from build123d import *

# Parameters (mm, degrees)
SKETCH1_W           = 480
SKETCH1_H           = 480
BOSS_EXTRUDE1_DEPTH = 190
BOSS_EXTRUDE1_DRAFT = 20
FILLET1_R           = 20
SKETCH2_R           = 120
BOSS_EXTRUDE2_DEPTH = 30
BOSS_EXTRUDE2_TAPER = 20
SHELL1_T            = -10
SCALE1_SCALE        = 0.5


with BuildPart() as part:
    # Sketch1 → Boss-Extrude1 (with draft: the straight prism first)
    with BuildSketch(Plane(origin=(0, 0, 0), x_dir=(1, 0, 0), z_dir=(0, 1, 0))):
        with Locations((240, -240)):
            Rectangle(SKETCH1_W, SKETCH1_H)
    extrude(amount=-BOSS_EXTRUDE1_DEPTH)
    # Boss-Extrude1: the draft: its side faces are tilted about the plane it starts from
    boss_extrude1_sides = [part.faces().sort_by_distance(p)[0] for p in [
        (0, -95, 240),
        (240, -95, 480),
        (480, -95, 240),
        (240, -95, 0),
    ]]
    draft(boss_extrude1_sides, Plane(origin=(0, 0, 0), x_dir=(1, 0, 0), z_dir=(0, 1, 0)), BOSS_EXTRUDE1_DRAFT)

    # Fillet1
    fillet1_edges = [part.edges().sort_by_distance(p)[0] for p in [
        (549.154344511, -190, 240),
        (240, -190, -69.154344511),
        (-69.154344511, -190, 240),
        (240, 0, 0),
        (480, 0, 240),
        (240, 0, 480),
        (0, 0, 240),
        (-34.577172255, -95, -34.577172255),
        (514.577172255, -95, -34.577172255),
        (514.577172255, -95, 514.577172255),
        (-34.577172255, -95, 514.577172255),
        (240, -190, 549.154344511),
    ]]
    fillet(fillet1_edges, radius=FILLET1_R)

    # Sketch2 → Boss-Extrude2 (add)
    with BuildSketch(Plane(origin=(0, 0, 0), x_dir=(1, 0, 0), z_dir=(0, 1, 0))):
        with Locations((240, -240)):
            Circle(SKETCH2_R)
    extrude(amount=BOSS_EXTRUDE2_DEPTH, taper=BOSS_EXTRUDE2_TAPER)

    # Shell1
    shell1_openings = [part.faces().sort_by_distance(p)[0] for p in [
        (240, 30, 240),
    ]]
    offset(amount=SHELL1_T, openings=shell1_openings, kind=Kind.INTERSECTION)


with BuildPart() as part_1:
    # Scale1: scaled about (0, 0, 0)
    add(part.part.scale(SCALE1_SCALE))


solid = part_1.part
Verification items for the finished model (mm, model axes). A direction names the side the tool comes from. Coordinates: 2 decimals unless noted, no trailing zeros. Write each loop counter-clockwise with the first axis right and the second up, starting at its lowest first coordinate (ties: lowest second). Pieces come first, ordered by that corner, then holes. Notation, with made-up numbers: M 45.5,19 L 103.5,19 A33 ccw 103.5,58 Z; hole C -29,6.25 d9. An arc over 180 degrees is marked long. Use a Markdown table: item, result.
Q1. Sectioned sample at C-C, the plane y = 6.5. Record the boundary of the cut face in (x, z).
Reply:
| item | result |
|---|---|
| outline | C 120,120 d115.27; hole C 120,120 d104.63 |
Q2. Sectioned sample at D-D, the plane x = 120. Record the boundary of the cut face in (y, z), plus the area to 3 significant figures.
Reply:
| item | result |
|---|---|
| outline | M -95,-20.3 A10 ccw -81.58,-29.69 L -6.58,-2.39 A10 ccw 0,7 L 0,60 L 15,65.46 L 15,70.78 L -5,63.5 L -5,7 A5 cw -8.29,2.3 L -83.29,-24.99 A5 cw -90,-20.3 L -90,260.3 A5 cw -83.29,264.99 L -8.29,237.7 A5 cw -5,233 L -5,176.5 L 15,169.22 L 15,174.54 L 0,180 L 0,233 A10 ccw -6.58,242.39 L -81.58,269.69 A10 ccw -95,260.3 Z |
| area | 3,170 mm² |
Q3. Go/stop test with flat-tipped pins: P1, Ø12, axis at x = 179, z = 85, coming from the +Y side; P2, Ø8, axis at y = -63.5, z = 14.5, coming from the -X side; P3, Ø5, axis at x = 82, y = -2.5, coming from the +Z side. Record where each tip stops, or that it passes through.
Reply:
| item | result |
|---|---|
| P1 | stops at y = 0 |
| P2 | stops at x = -24.57 |
| P3 | stops at z = 241.66 |
Q4. Sectioned sample at A-A, the plane z = 45. Record the boundary of the cut face in (x, y), plus the area to 3 significant figures.
Reply:
| item | result |
|---|---|
| outline | M -29.69,-81.58 A10 ccw -20.3,-95 L 260.3,-95 A10 ccw 269.69,-81.58 L 242.39,-6.58 A10 ccw 233,0 L 7,0 A10 ccw -2.39,-6.58 Z; hole M -24.99,-83.29 A5 ccw -20.3,-90 L 260.3,-90 A5 ccw 264.99,-83.29 L 237.7,-8.29 A5 ccw 233,-5 L 7,-5 A5 ccw 2.3,-8.29 Z |
| area | 3,570 mm² |
Q5. Thickness scan on line 1 (Y direction, x = 179.5, z = 178.5); line 2 (Z direction, x = 203, y = -36.5); line 3 (Z direction, x = 140.5, y = -89). Record the ranges inside material, lowest first.
Reply:
| item | result |
|---|---|
| line 1 | y = -95 to -90, -5 to 0 |
| line 2 | z = -13.28 to -7.96, 247.96 to 253.28 |
| line 3 | z = -29.46 to -23.3, 263.3 to 269.46 |
Q6. Draft check along Z on faces 1 (the face through (-15.85, -43.55, 121.96)), 2 (the face through (-13.2, -43.45, 253.05)), 3 (the face through (-24.43, -87.81, 118.04)). Enter one of: +Z half, -Z half, draft (parallel to the pull), parting line (faces both ways), or undercut.
Reply:
| item | result |
|---|---|
| face 1 | draft |
| face 2 | +Z half |
| face 3 | undercut |
Q7. Set-up check for faces 4 (the face through (121.96, -87.81, 264.43)), 5 (the face through (118, -95, 118)): record each of +Z, -Z, +X, -X, +Y, -Y from which the full face is reachable in a straight line by a thin tool's end or side.
Reply:
| item | result |
|---|---|
| face 4 | none |
| face 5 | +Z, -Z, +X, -X, -Y |
Q8. Sectioned sample at B-B, the plane x = 27.5. Record the boundary of the cut face in (y, z), plus the area to 3 significant figures.
Reply:
| item | result |
|---|---|
| outline | M -95,-20.3 A10 ccw -81.58,-29.69 L -6.58,-2.39 A10 ccw 0,7 L 0,233 A10 ccw -6.58,242.39 L -81.58,269.69 A10 ccw -95,260.3 Z; hole M -90,-20.3 A5 ccw -83.29,-24.99 L -8.29,2.3 A5 ccw -5,7 L -5,233 A5 ccw -8.29,237.7 L -83.29,264.99 A5 ccw -90,260.3 Z |
| area | 3,570 mm² |
